from build123d import *

# Parameters (mm, degrees)
SKETCH1_R           = 27.94
BOSS_EXTRUDE1_DEPTH = 114.3
SKETCH2_W           = 28.65102891
SKETCH2_H           = 3.175
SKETCH3_R           = 3.175
OUTLET_DEPTH        = 25.4
SKETCH4_W           = 50.8
SKETCH4_H           = 15.24


with BuildPart() as part:
    # Sketch1 → Boss-Extrude1 (new body)
    with BuildSketch(Plane(origin=(0, 0, 0), x_dir=(1, 0, 0), z_dir=(0, 1, 0))):
        with Locations(Location((0, 0, 0), (0, 0, 270))):
            Circle(SKETCH1_R)
    extrude(amount=BOSS_EXTRUDE1_DEPTH)

    # Sketch2 → inlet (revolve, cut)
    with BuildSketch(Plane.XY):
        with Locations((-29.319058082, 26.9875)):
            Rectangle(SKETCH2_W, SKETCH2_H)
    revolve(axis=Axis((-14.993543627, 25.4, 0), (-1, 0, 0)), mode=Mode.SUBTRACT)

    # Sketch3 → outlet (cut)
    with BuildSketch(Plane.XZ):
        with Locations(Location((0, 0, 0), (0, 0, 270))):
            Circle(SKETCH3_R)
    extrude(amount=-OUTLET_DEPTH, mode=Mode.SUBTRACT)

    # Sketch4 → Revolve1 (revolve)
    with BuildSketch(Plane.XY, mode=Mode.PRIVATE) as revolve1_sk:
        with Locations((-25.4, 76.2)):
            Rectangle(SKETCH4_W, SKETCH4_H)
    revolve(revolve1_sk.sketch.rotate(Axis((-50.8, 68.58, 0), (1, 0, 0)), 90), axis=Axis((-50.8, 68.58, 0), (1, 0, 0)))

    # Sketch6 → 1/2 NPT Tapped Hole1 (revolve, cut)
    with BuildSketch(Plane(origin=(-50.8, 68.58, 0), x_dir=(0, 0, 1), z_dir=(0, 1, 0))):
        Polygon((0, 0), (0, 27.970543693), (8.9281, 22.606), (8.9281, 13.462), (10.280678542, 13.462), (10.6647361, 0.635), (11.2997361, 0), align=None)
    revolve(axis=Axis((-57.15, 68.58, 0), (1, 0, 0)), mode=Mode.SUBTRACT)


solid = part.part
Verification items for the finished model (mm, model axes). A direction names the side the tool comes from. Give positions to 0.01 mm unless a question says otherwise; leave off trailing zeros. Write each loop counter-clockwise with the first axis right and the second up, starting at its lowest first coordinate (ties: lowest second). Pieces come first, ordered by that corner, then holes. Notation, with made-up numbers: M 68.25,30.5 L 107.25,30.5 A6 ccw 107.25,34.5 Z; hole C 76,-21.75 d6. An arc over 180 degrees is marked long. Put each result on its own line as item: value. Start each with the question number.
1. Section check A-A (x = 0). Record the cut outline in (y, z) (3 decimals).
2. Draft check along Y on faces 4 (the face through (-36.92, 82.1, 7.03)), 5 (the face through (-43.841, 77.873, 4.834)), 6 (the face through (-50.8, 57, 0)). Enter one of: +Y half, -Y half, draft (parallel to the pull), parting line (faces both ways), or undercut.
3. Section check D-D (x = -35.5). Record the cut outline in (y, z).
4. Section check C-C (y = 95.5). Record the cut outline in (x, z), and give its area (3 significant figures).
5. Section check B-B (z = -13). Record the cut outline in (x, y).
6. Set-up check for faces 1 (the face through (-14.994, 25, 0)), 2 (the face through (0, 25.4, 0)), 3 (the face through (-6, 0, 0)): record each of +Z, -Z, +X, -X, +Y, -Y from which the full face is reachable in a straight line by a thin tool's end or side.
7. Scan lines: line 1 along Y through (x, z) = (-31.5, 0); line 2 along X through (y, z) = (16, 0) (3 decimals); line 3 along Z through (x, y) = (-33, 68). Record each from-to range of solid material in increasing order. Write a range as [from, to].
8. Go/stop test with flat-tipped pins: pin 1 Ø12 at (y, z) = (39, -9) entering from -X; pin 2 Ø8.5 at (y, z) = (25.4, 0) entering from -X; pin 3 Ø6 at (x, y) = (3.5, 48) entering from -Z. Record where each tip stops, or that it passes through.
Answer list:
1. outline: M 0,-27.94 L 114.3,-27.94 L 114.3,27.94 L 0,27.94 L 0,3.175 L 25.4,3.175 L 25.4,-3.175 L 0,-3.175 Z
2. face 4: parting line
2. face 5: undercut
2. face 6: draft
3. outline: C 68.58,0 d30.48; hole C 68.58,0 d17.86
4. outline: C 0,0 d55.88
4. area: 2,450 mm2
5. outline: M -50.8,60.63 L -24.73,60.63 L -24.73,0 L 24.73,0 L 24.73,114.3 L -24.73,114.3 L -24.73,76.53 L -50.8,76.53 Z
6. face 1: -X
6. face 2: -Y
6. face 3: +Z, -Z, +X, -X, -Y
7. line 1: [53.34, 59.65], [77.51, 83.82]
7. line 2: [-27.94, -3.175], [3.175, 27.94]
7. line 3: [-15.23, -8.91], [8.91, 15.23]
8. pin 1: x = -27.78
8. pin 2: x = -27.94
8. pin 3: z = -27.94
